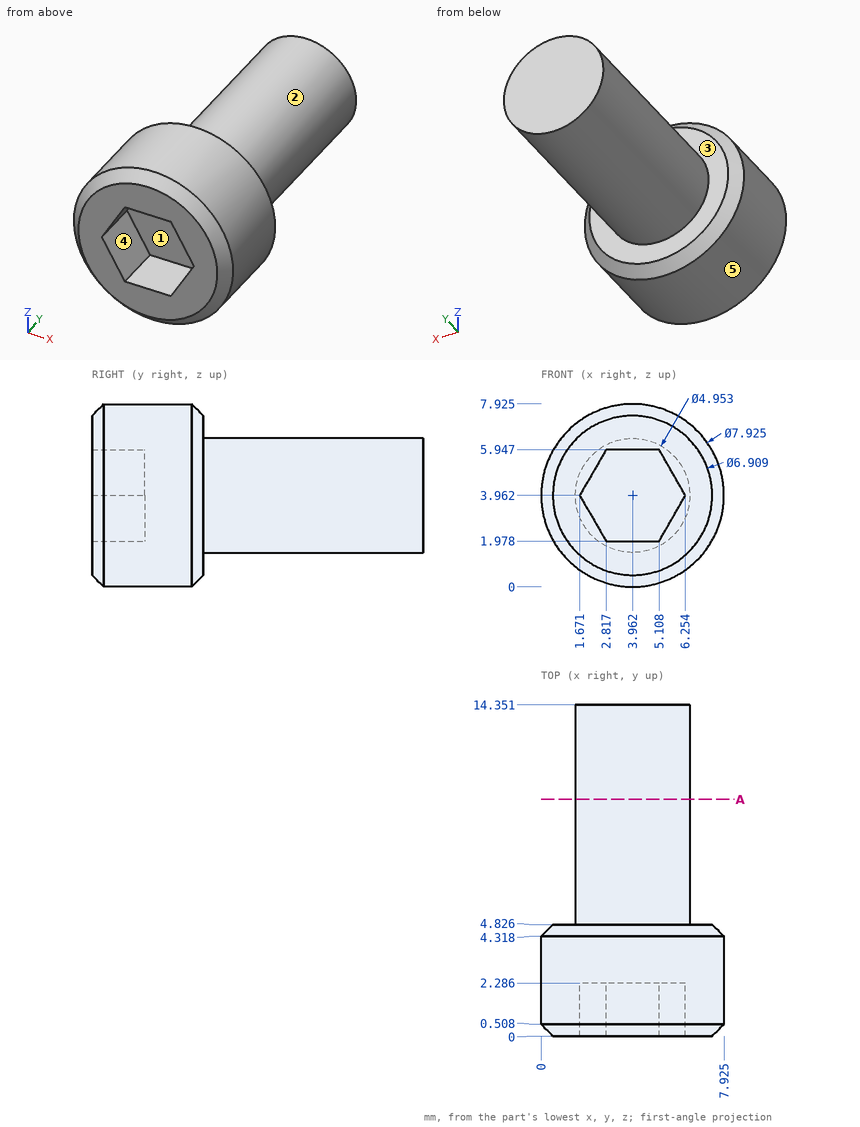
Here's the drawing with two shaded views (mm, measured from the low corner). I have some questions. A direction names the side the tool comes from. Coordinates: 2 decimals unless noted, no trailing zeros. Write each loop counter-clockwise with the first axis right and the second up, starting at its lowest first coordinate (ties: lowest second). Pieces come first, ordered by that corner, then holes. Notation, with made-up numbers: (27.25, -27.75) -> (37.25, -27.75) arc R29 cw to (37.25, -3.75) -> close; hole circle Ø1 at (55.25, 8). An arc over 180 degrees is marked (long way). Answer as CSV lines item,"result".
1) Will these pins go through, and if not, where does the flat tip stop? P1, Ø2, axis at x = 1.5, y = 4, coming from the -Z side; P2, Ø2, axis at y = 8.5, z = 4.5, coming from the -X side; P3, Ø0.7, axis at x = 4.5, y = 1.5, coming from the +Z side.
Check result:
P1,"z = 0.28"
P2,"x = 1.49"
P3,"z = 7.92"
2) If I drill on line 1 (Y direction, x = 3.5, z = 3.75); line 2 (Y direction, x = 5.75, z = 6.25); line 3 (X direction, y = 1, z = 5) (1 decimal), over which ranges is the centre line in solid material (lowest first)? Write a range as from..to.
Check result:
line 1,"2.29..14.35"
line 2,"0..4.83"
line 3,"0.1..2.3, 5.7..7.8"
3) On a 3-axis mill with a long thin cutter (end or side, diameter ignored), from which of +Z, -Z, +X, -X, +Y, -Y can I reach the whole of each face in a straight line? I mean the marked faces 4 and 5. Say none if no direction works.
Check result:
face 4,"-Y"
face 5,"+Y, -Y"
4) If we mould it in two halves opening along Z, with no side actions, what happens to the marked faces 1, 2 and 3? For each: +Z half, -Z half, draft (parallel to the pull), parting line (faces both ways), or undercut.
Check result:
face 1,"undercut"
face 2,"parting line"
face 3,"draft"
5) If we section it at A-A on y = 10.25: Please give me the cut outline in (x, z), then the cut area to 3 significant figures.
Check result:
outline,"circle Ø4.95 at (3.96, 3.96)"
area,"19.3 mm²"
